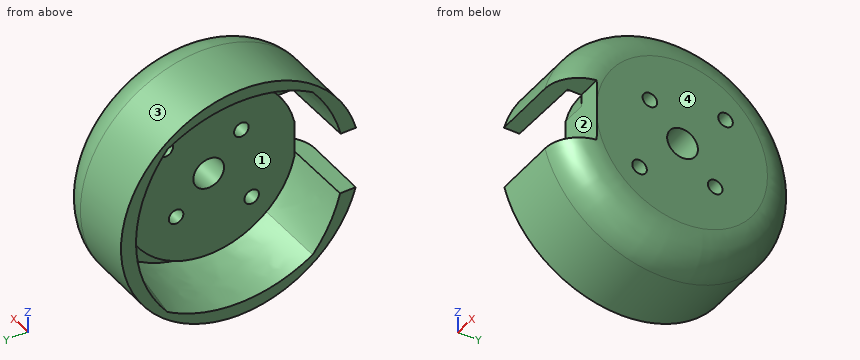
```python
from build123d import *

# Parameters (mm, degrees)
SKETCH1_R           = 24.584865892
BOSS_EXTRUDE4_DEPTH = 20
SKETCH5_R           = 17.9
BOSS_EXTRUDE5_DEPTH = 5
SKETCH6_R           = 1.5
SKETCH6_R_2         = 3.162859367
CUT_EXTRUDE1_DEPTH  = 10
FILLET1_R           = 7
SKETCH8_W           = 13
SKETCH8_H           = 8.974684843
CUT_EXTRUDE2_DEPTH  = 30


with BuildPart() as part:
    # Sketch1 → Boss-Extrude4 (new body)
    with BuildSketch(Plane(origin=(0, 0, 0), x_dir=(0, 0, -1), z_dir=(1, 0, 0))):
        with Locations((69.470275966, 107.4)):
            Circle(SKETCH1_R)
    extrude(amount=BOSS_EXTRUDE4_DEPTH)

    # Cut-Loft1: read off the stored shape, not the designer's step
    # Cut-Loft1: loft between two sections, ruled curve by curve
    cut_loft1_from = [
        Edge.make_bspline([(0, 122.421030793, -51.5998214), (0, 121.403963567, -50.977061653), (0, 120.31454314, -50.395752434), (0, 118.005938422, -49.358232659), (0, 116.786749472, -48.902260973), (0, 114.249384519, -48.15409937), (0, 112.931336418, -47.862145319), (0, 110.241321726, -47.469427252), (0, 108.869602219, -47.368811755), (0, 106.125867826, -47.368811755), (0, 104.754148319, -47.469427252), (0, 102.064133627, -47.862145319), (0, 100.746085526, -48.15409937), (0, 98.208720572, -48.902260973), (0, 96.989531623, -49.358232659), (0, 94.680926905, -50.395752434), (0, 93.591506478, -50.977061653), (0, 92.574439252, -51.5998214)], [0, 0, 0, 0, 0.125, 0.125, 0.25, 0.25, 0.375, 0.375, 0.5, 0.5, 0.625, 0.625, 0.75, 0.75, 0.875, 0.875, 1, 1, 1, 1], 3),
        Edge.make_bspline([(0, 92.574439252, -51.5998214), (0, 91.688670965, -52.66973324), (0, 90.833868812, -53.859032932), (0, 89.270225328, -56.474339023), (0, 88.562039976, -57.900649218), (0, 87.380791607, -60.949300184), (0, 86.90857847, -62.571462387), (0, 86.269439046, -65.928597857), (0, 86.103133633, -67.662819685), (0, 86.103133633, -71.132277338), (0, 86.269439046, -72.866499165), (0, 86.90857847, -76.223634636), (0, 87.380791607, -77.845796839), (0, 88.562039976, -80.894447804), (0, 89.270225328, -82.320757999), (0, 90.833868812, -84.93606409), (0, 91.688670965, -86.125363783), (0, 92.574439252, -87.195275623)], [0, 0, 0, 0, 0.125, 0.125, 0.25, 0.25, 0.375, 0.375, 0.5, 0.5, 0.625, 0.625, 0.75, 0.75, 0.875, 0.875, 1, 1, 1, 1], 3),
        Edge.make_bspline([(0, 122.421030793, -87.195275623), (0, 123.30679908, -86.125363783), (0, 124.161601233, -84.93606409), (0, 125.725244717, -82.320757999), (0, 126.433430069, -80.894447804), (0, 127.614678438, -77.845796839), (0, 128.086891575, -76.223634636), (0, 128.726030999, -72.866499165), (0, 128.892336412, -71.132277338), (0, 128.892336412, -67.662819685), (0, 128.726030999, -65.928597857), (0, 128.086891575, -62.571462387), (0, 127.614678438, -60.949300184), (0, 126.433430069, -57.900649218), (0, 125.725244717, -56.474339023), (0, 124.161601233, -53.859032932), (0, 123.30679908, -52.66973324), (0, 122.421030793, -51.5998214)], [0, 0, 0, 0, 0.125, 0.125, 0.25, 0.25, 0.375, 0.375, 0.5, 0.5, 0.625, 0.625, 0.75, 0.75, 0.875, 0.875, 1, 1, 1, 1], 3),
        Edge.make_bspline([(0, 92.574439252, -87.195275623), (0, 93.591506478, -87.818035369), (0, 94.680926905, -88.399344588), (0, 96.989531623, -89.436864364), (0, 98.208720572, -89.89283605), (0, 100.746085526, -90.640997653), (0, 102.064133627, -90.932951704), (0, 104.754148319, -91.325669771), (0, 106.125867826, -91.426285268), (0, 108.869602219, -91.426285268), (0, 110.241321726, -91.325669771), (0, 112.931336418, -90.932951704), (0, 114.249384519, -90.640997653), (0, 116.786749472, -89.89283605), (0, 118.005938422, -89.436864364), (0, 120.31454314, -88.399344588), (0, 121.403963567, -87.818035369), (0, 122.421030793, -87.195275623)], [0, 0, 0, 0, 0.125, 0.125, 0.25, 0.25, 0.375, 0.375, 0.5, 0.5, 0.625, 0.625, 0.75, 0.75, 0.875, 0.875, 1, 1, 1, 1], 3),
    ]
    cut_loft1_to = [
        Edge.make_bspline([(15, 121.083565639, -53.151068005), (15, 120.209787037, -52.418409479), (15, 119.250887023, -51.73451628), (15, 117.180423625, -50.51390478), (15, 116.06885476, -49.977467502), (15, 113.729261674, -49.097277381), (15, 112.501387925, -48.753802027), (15, 109.982206911, -48.291780772), (15, 108.691190331, -48.173409599), (15, 106.108809669, -48.173409599), (15, 104.817793089, -48.291780772), (15, 102.298612075, -48.753802027), (15, 101.070738326, -49.097277381), (15, 98.73114524, -49.977467502), (15, 97.619576375, -50.51390478), (15, 95.549112977, -51.73451628), (15, 94.590212963, -52.418409479), (15, 93.716434361, -53.151068005)], [0, 0, 0, 0, 0.125, 0.125, 0.25, 0.25, 0.375, 0.375, 0.5, 0.5, 0.625, 0.625, 0.75, 0.75, 0.875, 0.875, 1, 1, 1, 1], 3),
        Edge.make_bspline([(15, 93.716434361, -53.151068005), (15, 92.674354023, -54.024846606), (15, 91.668704432, -55.039081505), (15, 89.829123863, -57.346029779), (15, 88.995964625, -58.639100564), (15, 87.606260661, -61.455866338), (15, 87.050715794, -62.979351249), (15, 86.29878706, -66.15903997), (15, 86.103133633, -67.814359733), (15, 86.103133633, -71.126192199), (15, 86.29878706, -72.781511962), (15, 87.050715794, -75.961200683), (15, 87.606260661, -77.484685594), (15, 88.995964625, -80.301451369), (15, 89.829123863, -81.594522153), (15, 91.668704432, -83.901470427), (15, 92.674354023, -84.915705326), (15, 93.716434361, -85.789483927)], [0, 0, 0, 0, 0.125, 0.125, 0.25, 0.25, 0.375, 0.375, 0.5, 0.5, 0.625, 0.625, 0.75, 0.75, 0.875, 0.875, 1, 1, 1, 1], 3),
        Edge.make_bspline([(15, 121.083565639, -85.789483927), (15, 122.125645977, -84.915705326), (15, 123.131295568, -83.901470427), (15, 124.970876137, -81.594522153), (15, 125.804035375, -80.301451369), (15, 127.193739339, -77.484685594), (15, 127.749284206, -75.961200683), (15, 128.50121294, -72.781511962), (15, 128.696866367, -71.126192199), (15, 128.696866367, -67.814359733), (15, 128.50121294, -66.15903997), (15, 127.749284206, -62.979351249), (15, 127.193739339, -61.455866338), (15, 125.804035375, -58.639100564), (15, 124.970876137, -57.346029779), (15, 123.131295568, -55.039081505), (15, 122.125645977, -54.024846606), (15, 121.083565639, -53.151068005)], [0, 0, 0, 0, 0.125, 0.125, 0.25, 0.25, 0.375, 0.375, 0.5, 0.5, 0.625, 0.625, 0.75, 0.75, 0.875, 0.875, 1, 1, 1, 1], 3),
        Edge.make_bspline([(15, 93.716434361, -85.789483927), (15, 94.590212963, -86.522142453), (15, 95.549112977, -87.206035652), (15, 97.619576375, -88.426647153), (15, 98.73114524, -88.96308443), (15, 101.070738326, -89.843274551), (15, 102.298612075, -90.186749905), (15, 104.817793089, -90.64877116), (15, 106.108809669, -90.767142333), (15, 108.691190331, -90.767142333), (15, 109.982206911, -90.64877116), (15, 112.501387925, -90.186749905), (15, 113.729261674, -89.843274551), (15, 116.06885476, -88.96308443), (15, 117.180423625, -88.426647153), (15, 119.250887023, -87.206035652), (15, 120.209787037, -86.522142453), (15, 121.083565639, -85.789483927)], [0, 0, 0, 0, 0.125, 0.125, 0.25, 0.25, 0.375, 0.375, 0.5, 0.5, 0.625, 0.625, 0.75, 0.75, 0.875, 0.875, 1, 1, 1, 1], 3),
    ]
    cut_loft1 = Solid(Shell([*[Face.make_surface_from_curves(cut_loft1_from[k], cut_loft1_to[k]) for k in range(4)], Face(Wire(cut_loft1_from)), Face(Wire(cut_loft1_to))]))
    add(cut_loft1, mode=Mode.SUBTRACT)

    # Sketch5 → Boss-Extrude5 (add)
    with BuildSketch(Plane.ZY.offset(-15)):
        with Locations(Location((-69.470275966, 107.4, 0), (0, 0, 180))):
            Circle(SKETCH5_R)
    extrude(amount=BOSS_EXTRUDE5_DEPTH)

    # Sketch6 → Cut-Extrude1 (cut)
    with BuildSketch(Plane.ZY.offset(-10)):
        with Locations((-60.753803406, 116.36119697)):
            Circle(SKETCH6_R)
        with Locations((-78.431472936, 98.68352744)):
            Circle(SKETCH6_R)
        with Locations((-76.310152592, 114.239876626)):
            Circle(SKETCH6_R)
        with Locations((-62.87512375, 100.804847784)):
            Circle(SKETCH6_R)
        with Locations((-69.592638171, 107.522362205)):
            Circle(SKETCH6_R_2)
    extrude(amount=-CUT_EXTRUDE1_DEPTH, mode=Mode.SUBTRACT)

    # Fillet1
    fillet1_edges = [part.edges().sort_by_distance(p)[0] for p in [
        (20, 107.4, -44.885410074),
    ]]
    fillet(fillet1_edges, radius=FILLET1_R)

    # Sketch8 → Cut-Extrude2 (cut)
    with BuildSketch(Plane(origin=(20, 0, 0), x_dir=(0, 0, -1), z_dir=(1, 0, 0))):
        with Locations((69.592638171, 85.435019783)):
            Rectangle(SKETCH8_W, SKETCH8_H)
    extrude(amount=-CUT_EXTRUDE2_DEPTH, mode=Mode.SUBTRACT)


solid = part.part
```
CAD build for the part. Positions are in the model's coordinates, mm. Face numbers are marked on the shaded views. Coordinates: 2 decimals unless noted, no trailing zeros. Use CSV: the item, a comma, the result in double quotes. Start each with the question number.
Q1. Probe probe 1 along Y at (x, z) = (13, -85); probe 2 along Z at (x, y) = (13.5, 101.5); probe 3 along Z at (x, y) = (14.5, 112.5). List the from-to ranges inside material, lowest first. Write a range as from..to.
Q2. Drop flat-ended pins along their axis: P1, Ø1.5, axis at x = 8, y = 115.5, coming from the +Z side; P2, Ø1.5, axis at y = 96.5, z = -51, coming from the +X side; P3, Ø3, axis at x = 6, y = 86.5, coming from the +Z side; P4, Ø5.5, axis at y = 107.52, z = -69.59, coming from the -X side. Give the stop position or say it passes through.
Q3. Two-plate mould, pull along Z, no slides. Class the marked faces 1, 2, 3 and 4: +Z half, -Z half, draft (parallel to the pull), parting line (faces both ways), or undercut.
Q4. Cut at A-A, the plane x = 12.25. State how many separate pieces and enclosed holes the cut face has, then the cut area to 3 significant figures.
Here are the results:
1,probe 1,"88.34..92.53, 98.5..116.3, 122.3..126.46"
1,probe 2,"-93.32..-90.02, -86.37..-64.2, -61.55..-52.57, -48.91..-45.62"
1,probe 3,"-93.35..-90.18, -86.63..-52.31, -48.76..-45.59"
2,P1,"z = -46.01"
2,P2,"x = 19.27"
2,P3,"z = -54.37"
2,P4,"through"
3,face 1,"undercut"
3,face 2,"undercut"
3,face 3,"parting line"
3,face 4,"draft"
4,separate pieces,"2"
4,enclosed holes,"5"
4,area,"1,350 mm2"
